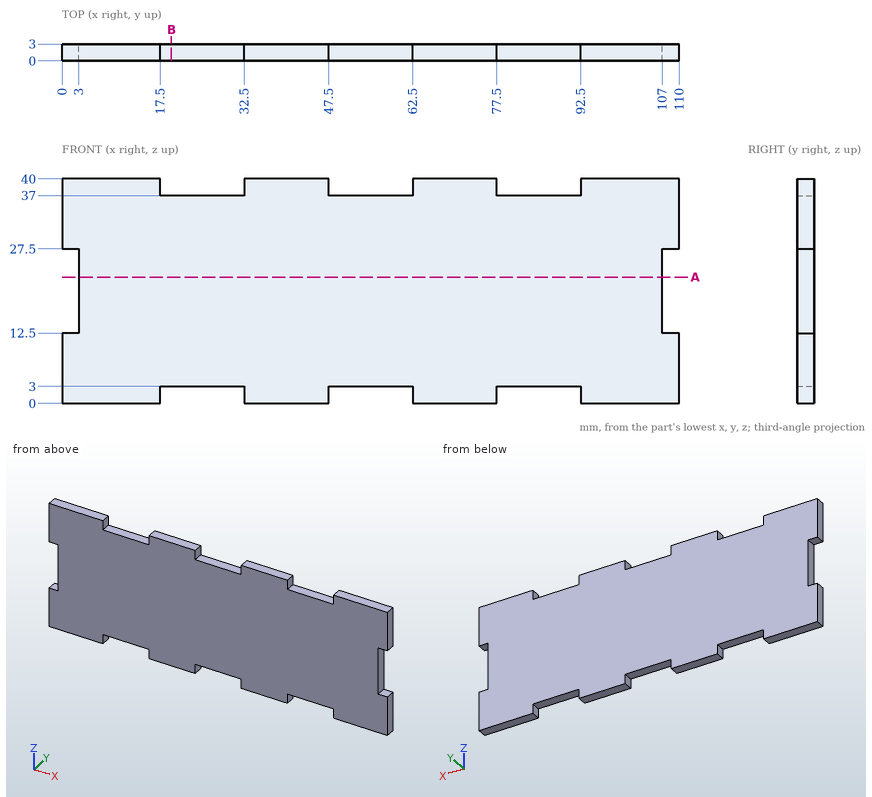
Check sheet for the drawn part. Datum: minimum x, y, z corner. Units: mm. Give positions to 0.01 mm unless a question says otherwise; leave off trailing zeros. Order: outer loops, then holes, each group sorted by start corner. A loop starts at its lowest first (then second) coordinate and runs counter-clockwise, first axis right, second up. Notation, with made-up numbers: (41, 57.25) - (71, 57.25) arc R25 ccw to (71, 79.25) - close; hole circle Ø2 at (68.5, 40). An arc over 180 degrees is marked (long way). Answer in a Markdown table with one row per item. Add a question column.
Q1. Cross-section at A-A, the plane z = 22.5. Enter the section's corners in (x, y), then the cut area to 3 significant figures.
Q2. Cross-section at B-B, the plane x = 19.5. Enter the section's corners in (y, z).
Q3. Material ranges on probe 1 along X at (y, z) = (0.2, 38.5); probe 2 along Z at (x, y) = (57.5, 0.1); probe 3 along X at (y, z) = (1.95, 22), recorded low to high. Write a range as from..to.
Q4. Gauge pin test, flat ends, axial feed: pin 1 (0.9 mm diameter, centred on x = 57.5, y = 1.5, fed in from -Z); pin 2 (1.5 mm diameter, centred on x = 55, y = 1, fed in from +Z); pin 3 (1.5 mm diameter, centred on y = 2, z = 16.5, fed in from +X). Record the tip position at first contact, or that the pin passes through.
Check values:
| question | item | result |
|---|---|---|
| 1 | outline | (3, 0) - (107, 0) - (107, 3) - (3, 3) - close |
| 1 | area | 312 mm^2 |
| 2 | outline | (0, 3) - (3, 3) - (3, 37) - (0, 37) - close |
| 3 | probe 1 | x = 0..17.5, 32.5..47.5, 62.5..77.5, 92.5..110 |
| 3 | probe 2 | z = 3..37 |
| 3 | probe 3 | x = 3..107 |
| 4 | pin 1 | stops at z = 3 |
| 4 | pin 2 | stops at z = 37 |
| 4 | pin 3 | stops at x = 107 |
